Geometry check sheet. Reference: the model listing, model coordinates, mm. A direction names the side the tool comes from. Coordinates: 2 decimals unless noted, no trailing zeros. Write each loop counter-clockwise with the first axis right and the second up, starting at its lowest first coordinate (ties: lowest second). Pieces come first, ordered by that corner, then holes. Notation, with made-up numbers: (41, 16) -> (79, 16) arc R21 ccw to (79, 42) -> close; hole circle Ø10 at (-11, -13). An arc over 180 degrees is marked (long way). Use a Markdown table: item, result.
```python
from build123d import *

# Parameters (mm, degrees)
SKETCH_1_R             = 18.5
SKETCH_1_W             = 35
SKETCH_1_H             = 23
EXTRUDE_1_DEPTH        = 3
CUT_EXTRUDE_START      = 1.5
SKETCH_1_3_R           = 20.5
SKETCH_1_3_R_2         = 18.5
CUT_EXTRUDE_1_DEPTH    = 1.5
FILLET_1_R             = 4.5
HOLE_WIZARD_M3_2_D     = 3.2
HOLE_WIZARD_M3_2_DEPTH = 12
HOLE_WIZARD_M4_1_D     = 4.3
SKETCH_1_4_R           = 4
CUT_EXTRUDE_2_DEPTH    = 287.041081094
EXTRUDE_2_DEPTH        = 6
FILLET_2_R             = 10
SKETCH_7_W             = 5
SKETCH_7_H             = 15
CUT_EXTRUDE_3_DEPTH    = 6


with BuildPart() as part:
    # ｽｹｯﾁ1 → ﾎﾞｽ - 押し出し1 (new, symmetric)
    with BuildSketch(Plane.XY):
        with BuildLine():
            Line((0, -29.5), (-255, -29.5))
            ThreePointArc((-255, -29.5), (-284.5, 0), (-255, 29.5))
            Line((-255, 29.5), (0, 29.5))
            ThreePointArc((0, 29.5), (29.5, 0), (0, -29.5))
        make_face()
        Circle(SKETCH_1_R, mode=Mode.SUBTRACT)
        with Locations((-255, 0)):
            Rectangle(SKETCH_1_W, SKETCH_1_H, mode=Mode.SUBTRACT)
    extrude(amount=EXTRUDE_1_DEPTH, both=True)

    # ｽｹｯﾁ1<3> → ｶｯﾄ - 押し出し1 (cut)
    with BuildSketch(Plane.XY.offset(CUT_EXTRUDE_START)):
        Circle(SKETCH_1_3_R)
        Circle(SKETCH_1_3_R_2, mode=Mode.SUBTRACT)
    extrude(amount=CUT_EXTRUDE_1_DEPTH, mode=Mode.SUBTRACT)

    # ﾌｨﾚｯﾄ1
    fillet_1_edges = [part.edges().sort_by_distance(p)[0] for p in [
        (-272.5, 11.5, 0),
        (-272.5, -11.5, 0),
        (-237.5, -11.5, 0),
        (-237.5, 11.5, 0),
    ]]
    fillet(fillet_1_edges, radius=FILLET_1_R)

    # M3 すきま穴2
    with Locations(Plane(origin=(-284.5, 0, 0), x_dir=(0, -1, 0), z_dir=(-1, 0, 0))):
        with Locations((0, 0)):
            Hole(HOLE_WIZARD_M3_2_D / 2, depth=HOLE_WIZARD_M3_2_DEPTH)

    # Hole Wizard M4 _1 (through all)
    with Locations(Plane(origin=(-192.444390405, 21, 3), x_dir=(1, 0, 0), z_dir=(0, 0, 1))):
        with Locations((0, 0), (100.122073915, 0), (100.122073915, -42), (0, -42)):
            Hole(HOLE_WIZARD_M4_1_D / 2)

    # ｽｹｯﾁ1<4> → ｶｯﾄ - 押し出し2 (cut, through all)
    with BuildSketch(Plane.XY):
        with Locations((-192.444390405, -21)):
            Circle(SKETCH_1_4_R)
        with Locations((-192.444390405, 21)):
            Circle(SKETCH_1_4_R)
        with Locations((-92.32231649, 21)):
            Circle(SKETCH_1_4_R)
        with Locations((-92.32231649, -21)):
            Circle(SKETCH_1_4_R)
    extrude(amount=CUT_EXTRUDE_2_DEPTH, mode=Mode.SUBTRACT)

    # ｽｹｯﾁ6 → ﾎﾞｽ - 押し出し2 (add)
    with BuildSketch(Plane.XY.offset(3)):
        with BuildLine():
            Line((0, 29.5), (30, 29.5))
            Line((30, 29.5), (30, -29.5))
            Line((30, -29.5), (0, -29.5))
            ThreePointArc((0, -29.5), (29.5, 0), (0, 29.5))
        make_face()
    extrude(amount=-EXTRUDE_2_DEPTH)

    # ﾌｨﾚｯﾄ2
    fillet_2_edges = [part.edges().sort_by_distance(p)[0] for p in [
        (30, 29.5, 0),
        (30, -29.5, 0),
    ]]
    fillet(fillet_2_edges, radius=FILLET_2_R)

    # ｽｹｯﾁ7 → ｶｯﾄ - 押し出し3 (cut)
    with BuildSketch(Plane.XY.offset(3)):
        with Locations((-286.030685235, 0)):
            Rectangle(SKETCH_7_W, SKETCH_7_H)
    extrude(amount=-CUT_EXTRUDE_3_DEPTH, mode=Mode.SUBTRACT)


solid = part.part
```
Item 1: Mould release check, pull along X, two halves, no side actions. Record for faces 4 (the cylindrical face through (26.99, 26.65, -0.04)), 5 (the flat face through (-125, 0, -3)), 6 (the flat face through (-191, -23, 0)), 7 (the flat face through (-283.531, -2, 0)): +X half, -X half, draft (parallel to the pull), parting line (faces both ways), or undercut.
Answer block:
| item | result |
|---|---|
| face 4 | +X half |
| face 5 | draft |
| face 6 | undercut |
| face 7 | -X half |
Item 2: Section check A-A on x = 0. Record the boundary of the cut face in (y, z).
Answer block:
| item | result |
|---|---|
| outline | (-29.5, -3) -> (-18.5, -3) -> (-18.5, 1.5) -> (-20.5, 1.5) -> (-20.5, 3) -> (-29.5, 3) -> close; (18.5, -3) -> (29.5, -3) -> (29.5, 3) -> (20.5, 3) -> (20.5, 1.5) -> (18.5, 1.5) -> close |
Item 3: Tool access check on faces 1 (the flat face through (-255, -11.5, 0)), 2 (the flat face through (-91, 19, 0)), 3 (the flat face through (-119, 29.5, 0)). Record the directions out of +Z, -Z, +X, -X, +Y, -Y that give a thin tool (end or side, any length) a straight path to the whole face; none if there is none.
Answer block:
| item | result |
|---|---|
| face 1 | +Z, -Z |
| face 2 | +Z |
| face 3 | +Z, -Z, +X, -X, +Y |
Item 4: Depth check by flat-ended pin: P1, Ø5, axis at x = -92.32, y = -21, coming from the -Z side; P2, Ø5, axis at x = -192.44, y = -21, coming from the +Z side; P3, Ø4, axis at x = -92.32, y = -21, coming from the +Z side; P4, Ø12.5, axis at x = -10, y = 9.5, coming from the +Z side. Enter the tip coordinate at first touch or a pass-through.
Answer block:
| item | result |
|---|---|
| P1 | stops at z = -3 |
| P2 | stops at z = 0 |
| P3 | passes through |
| P4 | stops at z = 1.5 |
Item 5: Thickness scan on L1, parallel to Y at x = 0, z = 2.25; L2, parallel to X at y = -21, z = 0.75; L3, parallel to X at y = -9.5, z = 1.6. Record the ranges inside material, lowest first. Write a range as [from, to].
Answer block:
| item | result |
|---|---|
| L1 | y = [-29.5, -20.5], [20.5, 29.5] |
| L2 | x = [-275.72, -196.44], [-188.44, -96.32], [-88.32, 29.89] |
| L3 | x = [-282.93, -271.74], [-238.26, -18.17], [18.17, 30] |
Item 6: Section check B-B on x = -261. Record the boundary of the cut face in (y, z), then the cut area to 3 significant figures.
Answer block:
| item | result |
|---|---|
| outline | (-28.88, -3) -> (-11.5, -3) -> (-11.5, 3) -> (-28.88, 3) -> close; (11.5, -3) -> (28.88, -3) -> (28.88, 3) -> (11.5, 3) -> close |
| area | 209 mm^2 |
